The figure shows three views and two pictorial views of one solid part (mm, origin at its lowest corner). Answer the questions. A direction names the side the tool comes from. Round coordinates to 2 decimals unless told otherwise and drop trailing zeros. Order: outer loops, then holes, each group sorted by start corner. A loop starts at its lowest first (then second) coordinate and runs counter-clockwise, first axis right, second up. Notation, with made-up numbers: M 64,21 L 110,21 A23 cw 110,55 Z; hole C 82.25,-32 d3. An arc over 180 degrees is marked long. Return JSON: item names as keys, results as strings.
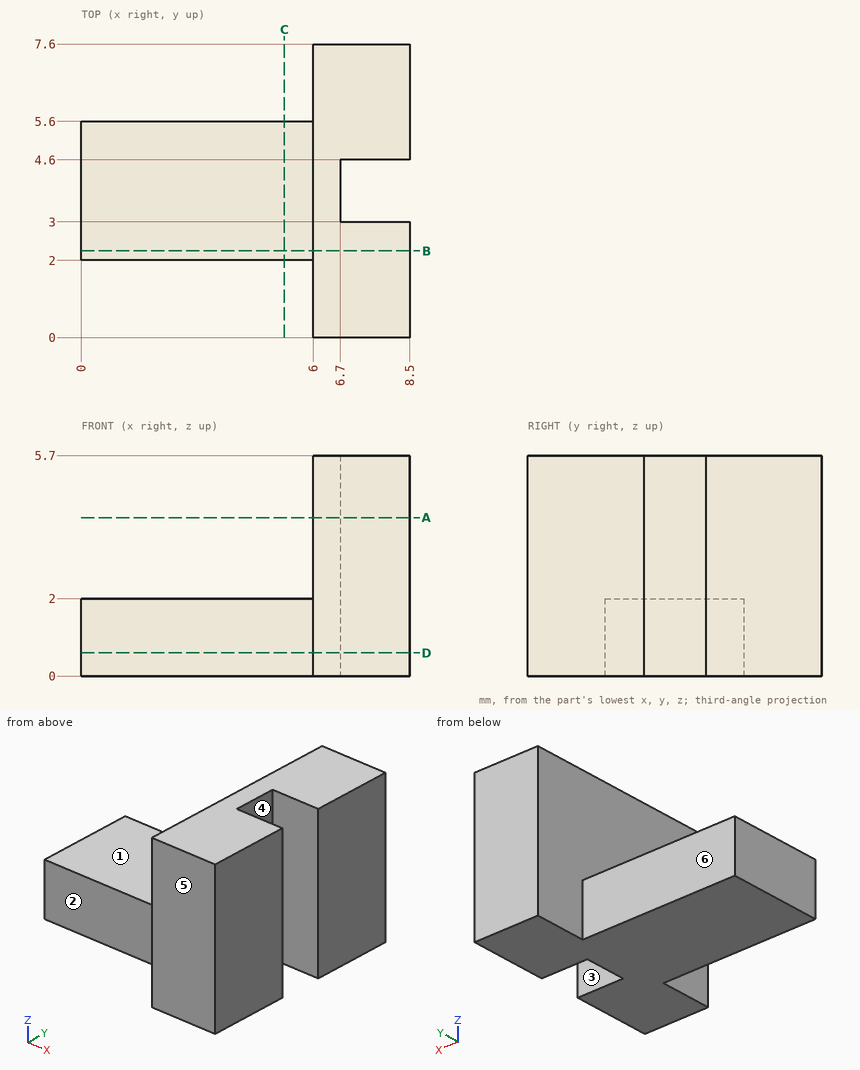
Item 1: Each of these flat-tipped pins is pushed along its axis until it touches: pin 1 (4 mm diameter, centred on x = 1.5, y = 4.5, fed in from +Z); pin 2 (2 mm diameter, centred on x = 3.5, z = 1, fed in from -Y); pin 3 (3 mm diameter, centred on x = 2.5, z = 2.5, fed in from +Y). Where does it stop, or does it pass through?
Output:
{"pin 1": "stops at z = 2", "pin 2": "stops at y = 2", "pin 3": "stops at y = 5.6"}
Item 2: Find section C-C (x = 5.25). Determine the outline of the cut face in (y, z), plus the area to 3 significant figures.
Output:
{"outline": "M 2,0 L 5.6,0 L 5.6,2 L 2,2 Z", "area": "7.20 mm^2"}
Item 3: Which of the six approach directions +Z, -Z, +X, -X, +Y, -Y give full straight-line access (tool end or side, diameter ignored) to the marked faces 4, 5 and 6?
Output:
{"face 4": "+Z, -Z, +X", "face 5": "+Z, -Z, +X, -X, -Y", "face 6": "+Z, -Z, -X, +Y"}
Item 4: Consider line 1 along X through (y, z) = (2.75, 3.9); line 2 along Y through (x, z) = (3.5, 0.75); line 3 along X through (y, z) = (3.5, 0.2). Determine where each line is inside the solid, lowest interval first. Write a range as [from, to].
Output:
{"line 1": "x = [6, 8.5]", "line 2": "y = [2, 5.6]", "line 3": "x = [0, 6.7]"}
Item 5: Find section B-B (y = 2.25). Determine the outline of the cut face in (x, z), plus the area to 4 significant figures.
Output:
{"outline": "M 0,0 L 8.5,0 L 8.5,5.7 L 6,5.7 L 6,2 L 0,2 Z", "area": "26.25 mm^2"}
Item 6: Find section A-A (z = 4.1). Determine the outline of the cut face in (x, y).
Output:
{"outline": "M 6,0 L 8.5,0 L 8.5,3 L 6.7,3 L 6.7,4.6 L 8.5,4.6 L 8.5,7.6 L 6,7.6 Z"}
Item 7: The mould has two halves that part along Y. Classify the marked faces 1, 2 and 3: pulls with the +Y half, pulls with the -Y half, needs draft (parallel to the pull), parting line crosses it, or undercut.
Output:
{"face 1": "needs draft", "face 2": "pulls with the -Y half", "face 3": "undercut"}
Item 8: Find section D-D (z = 0.6). Determine the outline of the cut face in (x, y), plus the area to 3 significant figures.
Output:
{"outline": "M 0,2 L 6,2 L 6,0 L 8.5,0 L 8.5,3 L 6.7,3 L 6.7,4.6 L 8.5,4.6 L 8.5,7.6 L 6,7.6 L 6,5.6 L 0,5.6 Z", "area": "37.7 mm^2"}
